Model file for the job. Use its own axes, mm. A direction names the side the tool comes from. Coordinates: 2 decimals unless noted, no trailing zeros. Order: outer loops, then holes, each group sorted by start corner. A loop starts at its lowest first (then second) coordinate and runs counter-clockwise, first axis right, second up. Notation, with made-up numbers: (81.5, 46.25) -> (106.5, 46.25) arc R7 cw to (106.5, 57.25) -> close; hole circle Ø2 at (66.25, -5). An arc over 180 degrees is marked (long way). Use CSV: the item, a comma, the result in double quotes. Start each with the question number.
(1) Cut at C-C on z = -4.5. Write the cut outline in (x, y).
(2) Cut at B-B on z = 0.5. Write the cut outline in (x, y).
(3) Tool access for faces 5 (the cylindrical face through (3.745, 7.473, -10.643)), 6 (the flat face through (-0.2, -8.3, 0)), 7 (the cylindrical face through (7.7, 2.42, -6.58)), 8 (the flat face through (3, 0, 6.35)): list every direction of +Z, -Z, +X, -X, +Y, -Y with a clear straight run to the whole face (end or side of a thin tool).
(4) Pull direction Y, two halves, no side cores. Call faces 1 (the cylindrical face through (-0.039, 3.683, 3.131)), 2 (the flat face through (0, 0, 0)), 3 (the flat face through (0, 0, -13.208)), 4 (the conical face through (4.64, 1.46, 3.2)): pulls with the +Y half, pulls with the -Y half, needs draft (parallel to the pull), parting line crosses it, or undercut.
(5) Cut at D-D on z = -10. Write the cut outline in (x, y), plus the area to 3 significant figures.
(6) Pin check, flat tips, straight feed: pin 1 Ø6 at (y, z) = (2, -1) entering from +X; pin 2 Ø8 at (x, z) = (-1, -4) entering from -Y; pin 3 Ø6 at (y, z) = (7, -3) entering from +X. Stop position of each tip, or through.
(7) Probe L1, parallel to Z at x = 11.75, y = -0.5; L2, parallel to X at y = -1.25, z = 5.25; L3, parallel to Z at x = 11, y = -4.25. List the from-to ranges inside material, lowest first.
```python
from build123d import *

# Parameters (mm, degrees)
F1_DEPTH    = 6.35
F2_R        = 12.6960047963
F2_R_2      = 8.0729751922
F3_DEPTH    = 5.08
F4_DEPTH    = 8.128
F5_R        = 12.7953112481
F5_R_2      = 1.3354653725
F5_R_3      = 8.0729751922
F6_DEPTH    = 5.08
F0_R        = 8.0645
F8_DEPTH    = 3.81
F9_S6_R     = 4.699
F9_T7_DEPTH = 39


# Not quite as in the source:
# - a fillet or chamfer that OpenCascade refuses, or shapes differently, is made with other operations: its cross-section is extruded or revolved along the edge and cut away or added


with BuildPart() as f1:
    # F0 (on Top) → F1 (new body)
    with BuildSketch(Plane.XY):
        with BuildLine():
            Line((-2.54, -2.8050532779), (-3.7699173874, -2.8050532779))
            ThreePointArc((-3.7699173874, -2.8050532779), (-0.0014195763, -4.6989997856), (3.7682218762, -2.8073305634))
            Line((3.7682218762, -2.8073305634), (2.54, -2.8073305634))
            Line((2.54, -2.8073305634), (2.54, -2.667))
            ThreePointArc((2.54, -2.667), (0, -3.683), (-2.54, -2.667))
            Line((-2.54, -2.667), (-2.54, -2.8050532779))
        make_face()
        with BuildLine():
            Line((2.54, 0), (2.54, -2.667))
            ThreePointArc((2.54, -2.667), (3.3852111456, -1.4508047767), (3.683, 0))
            ThreePointArc((3.683, 0), (3.3852111456, 1.4508047767), (2.54, 2.667))
            Line((2.54, 2.667), (2.54, 0))
        make_face()
        with BuildLine():
            Line((2.54, -2.8073305634), (3.7682218762, -2.8073305634))
            Line((3.7682218762, -2.8073305634), (3.7682218762, 2.667))
            Line((3.7682218762, 2.667), (2.54, 2.667))
            ThreePointArc((2.54, 2.667), (3.3852111456, 1.4508047767), (3.683, 0))
            ThreePointArc((3.683, 0), (3.3852111456, -1.4508047767), (2.54, -2.667))
            Line((2.54, -2.667), (2.54, -2.8073305634))
        make_face()
        with BuildLine():
            ThreePointArc((3.7682218762, -2.8073305634), (4.460239657, -1.4788046531), (4.699, 0))
            ThreePointArc((4.699, 0), (-1.4774571392, 4.460686203), (-3.7699173874, -2.8050532779))
            Line((-3.7699173874, -2.8050532779), (-3.7699173874, 2.667))
            Line((-3.7699173874, 2.667), (-2.54, 2.667))
            ThreePointArc((-2.54, 2.667), (0, 3.683), (2.54, 2.667))
            Line((2.54, 2.667), (3.7682218762, 2.667))
            Line((3.7682218762, 2.667), (3.7682218762, -2.8073305634))
        make_face()
        with BuildLine():
            Line((-3.7699173874, 2.667), (-3.7699173874, -2.8050532779))
            Line((-3.7699173874, -2.8050532779), (-2.54, -2.8050532779))
            Line((-2.54, -2.8050532779), (-2.54, -2.667))
            ThreePointArc((-2.54, -2.667), (-3.683, 0), (-2.54, 2.667))
            Line((-2.54, 2.667), (-3.7699173874, 2.667))
        make_face()
        with BuildLine():
            ThreePointArc((-2.54, 2.667), (-3.683, 0), (-2.54, -2.667))
            Line((-2.54, -2.667), (-2.54, 0))
            Line((-2.54, 0), (-2.54, 2.667))
        make_face()
    extrude(amount=F1_DEPTH)



with BuildPart() as f3:
    # F2 (on Top) → F3 (new body)
    with BuildSketch(Plane.XY):
        Circle(F2_R)
        Circle(F2_R_2, mode=Mode.SUBTRACT)
    extrude(amount=-F3_DEPTH)


with BuildPart() as f1_1:
    add(f1.part)

    add(f3.part)  # F4 merges F3
    # F2 (on Top) → F4 (join)
    with BuildSketch(Plane.XY):
        Circle(F2_R_2)
    extrude(amount=-F4_DEPTH)

    # F5 (on face) → F6 (join)
    with BuildSketch(Plane(origin=(0, 0, -8.128), x_dir=(1, 0, 0), z_dir=(0, 0, -1))):
        Circle(F5_R)
        with Locations((3.9191520773, -8.7972320383)):
            Circle(F5_R_2, mode=Mode.SUBTRACT)
        Circle(F5_R_3, mode=Mode.SUBTRACT)
        Circle(F5_R_3)
    extrude(amount=F6_DEPTH)

    # F7: fillet of radius 5.08 on 2 edges, made by hand

    # F7_s1 → F7_t2 (revolve, cut)
    with BuildSketch(Plane.XZ):
        with BuildLine():
            ThreePointArc((12.7953112481, -13.1953934624), (11.4317162877, -9.7320520727), (8.0729751922, -8.128))
            Line((8.0729751922, -8.128), (12.7953112481, -8.128))
            Line((12.7953112481, -8.128), (12.7953112481, -13.1953934624))
        make_face()
    revolve(axis=Axis((0, 0, -8.128), (0, 0, -1)), mode=Mode.SUBTRACT)

    # F7_s3 → F7_t4 (revolve, cut)
    with BuildSketch(Plane.XZ):
        with BuildLine():
            ThreePointArc((8.0729751922, -5.08), (11.366192099, -3.4473275256), (12.6960047963, -0.0205950886))
            Line((12.6960047963, -0.0205950886), (12.6960047963, -5.08))
            Line((12.6960047963, -5.08), (8.0729751922, -5.08))
        make_face()
    revolve(axis=Axis((0, 0, -5.08), (0, 0, 1)), mode=Mode.SUBTRACT)

    # F0 (on Top) → F8 (join)
    with BuildSketch(Plane.XY):
        Circle(F0_R)
        with BuildLine():
            ThreePointArc((-3.7699173874, -2.8050532779), (-1.4774571392, 4.460686203), (4.699, 0))
            ThreePointArc((4.699, 0), (4.460239657, -1.4788046531), (3.7682218762, -2.8073305634))
            ThreePointArc((3.7682218762, -2.8073305634), (-0.0014195763, -4.6989997856), (-3.7699173874, -2.8050532779))
        make_face(mode=Mode.SUBTRACT)
    extrude(amount=F8_DEPTH)

    # F9: chamfer of 3.81 on 1 edges, made by hand


with BuildPart() as f9_tool2:
    # F9_s3 → F9_t4 (revolve)
    with BuildSketch(Plane.XZ):
        with BuildLine():
            Line((8.1722630735, -0.1077630735), (4.1467369265, 3.9177630735))
            Line((4.1467369265, 3.9177630735), (4.1467369265, 3.9939630735))
            ThreePointArc((4.1467369265, 3.9939630735), (6.1056184633, 3.8862), (8.0645, 3.8862))
            Line((8.0645, 3.8862), (8.1407, 3.81))
            ThreePointArc((8.1407, 3.81), (8.1407, 1.8511184633), (8.2484630735, -0.1077630735))
            Line((8.2484630735, -0.1077630735), (8.1722630735, -0.1077630735))
        make_face()
    revolve(axis=Axis((0, 0, 3.81), (0, 0, 1)))

    split(bisect_by=Plane.XY, keep=Keep.TOP)

    # F9_s6 → F9_t7 (cut, symmetric)
    with BuildSketch(Plane.XY.offset(2.8)):
        Circle(F9_S6_R)
    extrude(amount=F9_T7_DEPTH, both=True, mode=Mode.SUBTRACT)


with BuildPart() as f1_2:
    add(f1_1.part)

    # F9_t1: cut F9_tool2
    add(f9_tool2.part, mode=Mode.SUBTRACT)


solid = f1_2.part
```
Outcome:
1,outline,"circle Ø20.02 at (0, 0)"
2,outline,"circle Ø15.13 at (0, 0); hole (-2.54, -2.67) arc R3.68 ccw to (2.54, -2.67) -> (2.54, 2.67) arc R3.68 ccw to (-2.54, 2.67) -> close"
3,face 5,"-Z"
3,face 6,"+Z"
3,face 7,"none"
3,face 8,"+Z, +X, -X, +Y, -Y"
4,face 1,"undercut"
4,face 2,"undercut"
4,face 3,"needs draft"
4,face 4,"parting line crosses it"
5,outline,"circle Ø23.33 at (0, 0); hole circle Ø2.67 at (3.92, 8.8)"
5,area,"422 mm2"
6,pin 1,"x = 12.7"
6,pin 2,"y = -12.7"
6,pin 3,"x = 11.69"
7,L1,"-13.21 to -10.12, -2.96 to 0"
7,L2,"-4.53 to -2.54, 2.54 to 4.53"
7,L3,"-13.21 to -10.17, -2.91 to 0"
